Can you work these out from the drawing? Everything is in mm from the part's minimum corner. Give positions to 0.01 mm unless a question says otherwise; leave off trailing zeros. Write each loop counter-clockwise with the first axis right and the second up, starting at its lowest first coordinate (ties: lowest second). Pieces come first, ordered by that corner, then holes. Notation, with made-up numbers: (47, 39.25) - (67, 39.25) arc R22 ccw to (67, 49.25) - close; hole circle Ø1 at (1.25, 71). An arc over 180 degrees is marked (long way). Write each question's results on one line, items separated by ' | '. Start each with the question number.
Item 1: Please list where these lines run through material, in increasing order: line 1 along Z through (x, y) = (59, 2.4); line 2 along X through (y, z) = (1.7, 112.5); line 3 along X through (y, z) = (2.25, 20) (3 decimals).
Item 2: Suppose I cut it at A-A on x = 7.5. List the corners of the cut face in (y, z) for me, then the cut area to 3 significant figures.
Item 3: Suppose I cut it at C-C on y = 1.45. Count the separate pieces of the cut face and the enclosed holes in it, then the cut area to 3 significant figures.
Item 4: Will this pin go through, and if not, where does the flat tip stop? P1, Ø2.5, axis at x = 42.965, z = 86, coming from the -Y side.
Item 5: Suppose I cut it at B-B on z = 112.5. List the corners of the cut face in (x, y) for me.
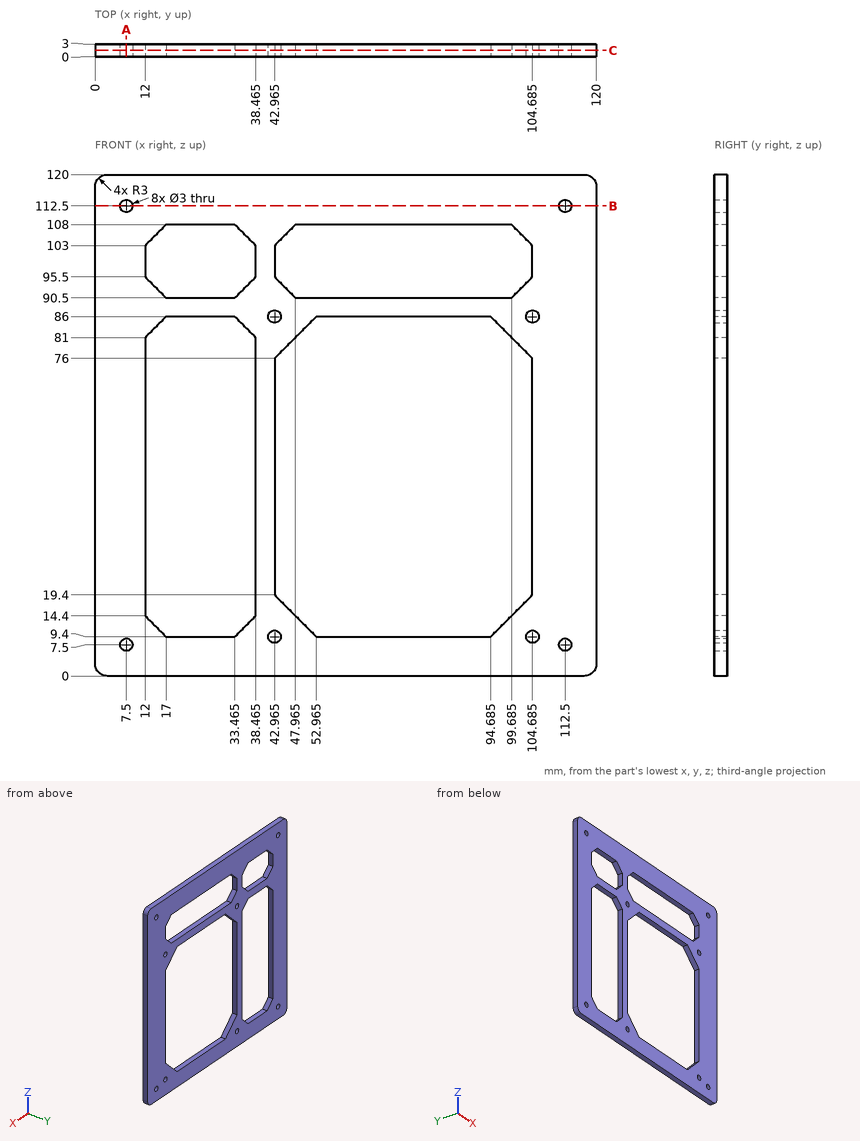
Checked values:
1) line 1: z = 0 to 9.4, 86 to 90.5, 108 to 120 | line 2: x = 0 to 6, 9 to 111, 114 to 120 | line 3: x = 0 to 12, 38.465 to 42.965, 104.685 to 120
2) outline: (0, 0) - (3, 0) - (3, 6) - (0, 6) - close; (0, 9) - (3, 9) - (3, 111) - (0, 111) - close; (0, 114) - (3, 114) - (3, 120) - (0, 120) - close | area: 342 mm^2
3) separate pieces: 1 | enclosed holes: 12 | area: 6,390 mm^2
4) P1: passes through
5) outline: (0, 0) - (6, 0) - (6, 3) - (0, 3) - close; (9, 0) - (111, 0) - (111, 3) - (9, 3) - close; (114, 0) - (120, 0) - (120, 3) - (114, 3) - close
